from build123d import *

# Parameters (mm, degrees)
BOX001_W               = 2
BOX001_H               = 10
BOX001_DEPTH           = 2
BOX001_PLACEMENT_ANGLE = 340
BOX_W                  = 2
BOX_H                  = 10
BOX_DEPTH              = 2
BOX_PLACEMENT_ANGLE    = 20


with BuildPart() as cub001:
    # Box001 → Box001 (new body)
    with BuildSketch(Plane.XY):
        with Locations((1, 5)):
            Rectangle(BOX001_W, BOX001_H)
    extrude(amount=BOX001_DEPTH)


with BuildPart() as cub001_1:
    # Box001 placement: moved
    add(cub001.part.moved(Location((0, 0.68, 0))).rotate(Axis((0, 0.68, 0), (0, 0, 1)), BOX001_PLACEMENT_ANGLE))


with BuildPart() as fusion:
    # Box → Box (new body)
    with BuildSketch(Plane.XY):
        with Locations((1, 5)):
            Rectangle(BOX_W, BOX_H)
    extrude(amount=BOX_DEPTH)


with BuildPart() as fusion_1:
    # Box placement: moved
    add(fusion.part.moved(Location((3.4, 0, 0))).rotate(Axis((3.4, 0, 0), (0, 0, 1)), BOX_PLACEMENT_ANGLE))

    # Fusion: union Cub001
    add(cub001_1.part)


solid = fusion_1.part
Model file for the job. Use its own axes, mm. A direction names the side the tool comes from. Give positions to 0.01 mm unless a question says otherwise; leave off trailing zeros. Loops run counter-clockwise (first coordinate to the right, second up) from the corner with the lowest first, then second, coordinate; pieces in that order, holes last.
1) Pull direction Y, two halves, no side cores. Call faces 1 (the flat face through (3.025, 8.991, 0.986)), 2 (the flat face through (3, 5, 0)), 3 (the flat face through (0.79, 7.17, 0.99)): +Y half, -Y half, draft (parallel to the pull), parting line (faces both ways), or undercut.
2) Saw through at D-D (y = 7). Write the cut outline in (x, z).
3) Saw through at B-B (z = 1). Write the cut outline in (x, y).
4) Flat gauge pin, fed straight in: pin 1 Ø1 at (x, y) = (2.5, 7) entering from -Z. Where does the tip first touch, or does it go through?
5) Saw through at C-C (y = 8.5). Write the cut outline in (x, z).
6) Wall check: line 1 (X direction, y = 9.25, z = 0.15); line 2 (X direction, y = 1.5, z = 0.4); line 3 (X direction, y = 7, z = 1.3). Give the ranges that are in metal, low to high.
7) Saw through at A-A (x = 4.45). Write the cut outline in (y, z), plus the area to 3 significant figures.
8) Tool access for faces 4 (the flat face through (0.78, 2.82, 0.99)), 5 (the flat face through (3.026, 1.029, 0.986)), 6 (the flat face through (2.255, 8.993, 0.986)), 7 (the flat face through (4.5, 7.2, 1)): list every direction of +Z, -Z, +X, -X, +Y, -Y with a clear straight run to the whole face (end or side of a thin tool).
Answer block:
1. face 1: +Y half
1. face 2: draft
1. face 3: undercut
2. outline: (0.85, 0) - (4.43, 0) - (4.43, 2) - (0.85, 2) - close
3. outline: (-0.02, 9.4) - (1.58, 5.01) - (0, 0.68) - (1.88, 0) - (2.64, 2.09) - (3.4, 0) - (5.28, 0.68) - (3.7, 5.01) - (5.3, 9.39) - (3.42, 10.08) - (2.64, 7.93) - (1.86, 10.08) - close
4. pin 1: stops at z = 0
5. outline: (0.31, 0) - (2.43, 0) - (2.43, 2) - (0.31, 2) - close; (2.85, 0) - (4.97, 0) - (4.97, 2) - (2.85, 2) - close
6. line 1: x = 0.03 to 2.16, 3.12 to 5.25
6. line 2: x = 0.3 to 2.43, 2.85 to 4.98
6. line 3: x = 0.85 to 4.43
7. outline: (0.38, 0) - (2.96, 0) - (2.96, 2) - (0.38, 2) - close; (7.06, 0) - (9.7, 0) - (9.7, 2) - (7.06, 2) - close
7. area: 10.4 mm2
8. face 4: +Z, -Z, -X
8. face 5: +Z, -Z, -Y
8. face 6: +Z, -Z, +Y
8. face 7: +Z, -Z, +X
